Geometry check sheet. Reference: the model listing, model coordinates, mm. A direction names the side the tool comes from. Coordinates: 2 decimals unless noted, no trailing zeros. Loops run counter-clockwise (first coordinate to the right, second up) from the corner with the lowest first, then second, coordinate; pieces in that order, holes last. Notation, with made-up numbers: M 48,55 L 52,55 A28 ccw 52,78 Z; hole C 62.5,-9.75 d3. An arc over 180 degrees is marked long. Use CSV: the item, a comma, the result in double quotes.
```python
from build123d import *

# Parameters (mm, degrees)
SKETCH_1_W          = 72
SKETCH_1_H          = 55
EXTRUDE_1_DEPTH     = 4
FILLET_1_R          = 2
CUT_EXTRUDE_1_REACH = 6
CUT_EXTRUDE_2_DEPTH = 2


with BuildPart() as part:
    # 草图1 → 凸台-拉伸1 (new body)
    with BuildSketch(Plane.XY):
        Rectangle(SKETCH_1_W, SKETCH_1_H)
    extrude(amount=EXTRUDE_1_DEPTH)

    # 圆角1
    fillet_1_edges = [part.edges().sort_by_distance(p)[0] for p in [
        (-36, 27.5, 2),
        (36, 27.5, 2),
        (36, -27.5, 2),
        (-36, -27.5, 2),
    ]]
    fillet(fillet_1_edges, radius=FILLET_1_R)

    # 草图2 → 切除-拉伸1 (cut, up to next)
    with BuildSketch(Plane.XY.offset(4), mode=Mode.PRIVATE) as cut_extrude_1_sk1:
        with BuildLine():
            Line((-31, 9.5), (-31, -9.5))
            ThreePointArc((-31, -9.5), (-27.485281374, -17.985281374), (-19, -21.5))
            Line((-19, -21.5), (19, -21.5))
            ThreePointArc((19, -21.5), (27.485281374, -17.985281374), (31, -9.5))
            Line((31, -9.5), (31, 9.5))
            ThreePointArc((31, 9.5), (27.485281374, 17.985281374), (19, 21.5))
            Line((19, 21.5), (-19, 21.5))
            ThreePointArc((-19, 21.5), (-27.485281374, 17.985281374), (-31, 9.5))
        make_face()
    cut_extrude_1_tool1 = extrude(cut_extrude_1_sk1.sketch, amount=-CUT_EXTRUDE_1_REACH, mode=Mode.PRIVATE) & part.part
    add(cut_extrude_1_tool1.solids().sort_by_distance((0, 0, 4))[0], mode=Mode.SUBTRACT)

    # 草图3 → 切除-拉伸2 (cut)
    with BuildSketch(Plane.XY.offset(4)):
        with BuildLine():
            Line((18.7, 24.3), (-18.7, 24.3))
            ThreePointArc((-18.7, 24.3), (-29.306601718, 19.906601718), (-33.7, 9.3))
            Line((-33.7, 9.3), (-33.7, -9.3))
            ThreePointArc((-33.7, -9.3), (-29.306601718, -19.906601718), (-18.7, -24.3))
            Line((-18.7, -24.3), (18.7, -24.3))
            ThreePointArc((18.7, -24.3), (29.306601718, -19.906601718), (33.7, -9.3))
            Line((33.7, -9.3), (33.7, 9.3))
            ThreePointArc((33.7, 9.3), (29.306601718, 19.906601718), (18.7, 24.3))
        make_face()
    extrude(amount=-CUT_EXTRUDE_2_DEPTH, mode=Mode.SUBTRACT)


solid = part.part
```
1. Section check C-C, the plane x = 4. Record the cut outline in (y, z).
The answers:
outline,"M -27.5,0 L -21.5,0 L -21.5,2 L -24.3,2 L -24.3,4 L -27.5,4 Z; M 21.5,0 L 27.5,0 L 27.5,4 L 24.3,4 L 24.3,2 L 21.5,2 Z"
2. Section check B-B, the plane z = 3.2. Record the cut outline in (x, y), plus the area to 3 significant figures.
The answers:
outline,"M -36,-25.5 A2 ccw -34,-27.5 L 34,-27.5 A2 ccw 36,-25.5 L 36,25.5 A2 ccw 34,27.5 L -34,27.5 A2 ccw -36,25.5 Z; hole M -33.7,-9.3 A15 ccw -18.7,-24.3 L 18.7,-24.3 A15 ccw 33.7,-9.3 L 33.7,9.3 A15 ccw 18.7,24.3 L -18.7,24.3 A15 ccw -33.7,9.3 Z"
area,"874 mm^2"
3. Release check for a two-part mould opening along X. For faces 1 (the cylindrical face through (-35.43, -26.9, 2.03)), 2 (the flat face through (0, -27.5, 2)), 3 (the cylindrical face through (-27.58, -17.89, 1.01)) record: +X half, -X half, draft (parallel to the pull), parting line (faces both ways), or undercut.
The answers:
face 1,"-X half"
face 2,"draft"
face 3,"undercut"
4. Section check A-A, the plane y = -4.5. Record the cut outline in (x, z).
The answers:
outline,"M -36,0 L -31,0 L -31,2 L -33.7,2 L -33.7,4 L -36,4 Z; M 31,0 L 36,0 L 36,4 L 33.7,4 L 33.7,2 L 31,2 Z"
5. Set-up check for faces 4 (the cylindrical face through (35.43, 26.9, 2.03)), 5 (the cylindrical face through (-27.39, 18.08, 1.01)), 6 (the flat face through (33.7, 0, 3)): record each of +Z, -Z, +X, -X, +Y, -Y from which the full face is reachable in a straight line by a thin tool's end or side.
The answers:
face 4,"+Z, -Z, +X, +Y"
face 5,"+Z, -Z"
face 6,"+Z"
6. Thickness scan on line 1 (Y direction, x = -19.5, z = 0.45); line 2 (Y direction, x = 0.5, z = 3.4); line 3 (X direction, y = 1, z = 3.4). Record the ranges inside material, lowest first. Write a range as [from, to].
The answers:
line 1,"[-27.5, -21.49], [21.49, 27.5]"
line 2,"[-27.5, -24.3], [24.3, 27.5]"
line 3,"[-36, -33.7], [33.7, 36]"
